Job drawing, mm, ordinate dimensions from the low corner. One solid piece. A direction names the side the tool comes from. Give positions to 0.01 mm unless a question says otherwise; leave off trailing zeros. Order: outer loops, then holes, each group sorted by start corner. A loop starts at its lowest first (then second) coordinate and runs counter-clockwise, first axis right, second up. Notation, with made-up numbers: M 14.25,70 L 28.25,70 A17 ccw 28.25,101 Z; hole C -13,87.5 d5. An arc over 180 degrees is marked long. Use CSV: the item, a comma, the result in double quotes. Start each with the question number.
Item 1: Wall check: line 1 along Z through (x, y) = (24, 6.25); line 2 along X through (y, z) = (16.5, 6.5); line 3 along Y through (x, z) = (31, 18.25). Give the ranges that are in metal, low to high.
Item 2: Band-saw the part on D-D on z = 12.5. Write the cut outline in (x, y), plus the area to 3 significant figures.
Item 3: Band-saw the part on A-A on x = 20. Write the cut outline in (y, z), plus the area to 3 significant figures.
Item 4: Two-plate mould, pull along X, no slides. Class the marked faces 1, 2 and 3: pulls with the +X half, pulls with the -X half, needs draft (parallel to the pull), parting line crosses it, or undercut.
Item 5: Which spindle directions (+Z, -Z, +X, -X, +Y, -Y) get a long thin tool onto all of the face, cutting with end or side? Do the marked faces 4 and 5. Say none if no direction does.
Item 6: Band-saw the part on B-B on z = 18. Write the cut outline in (x, y).
Item 7: Band-saw the part on C-C on y = 9.5. Write the cut outline in (x, z), plus the area to 3 significant figures.
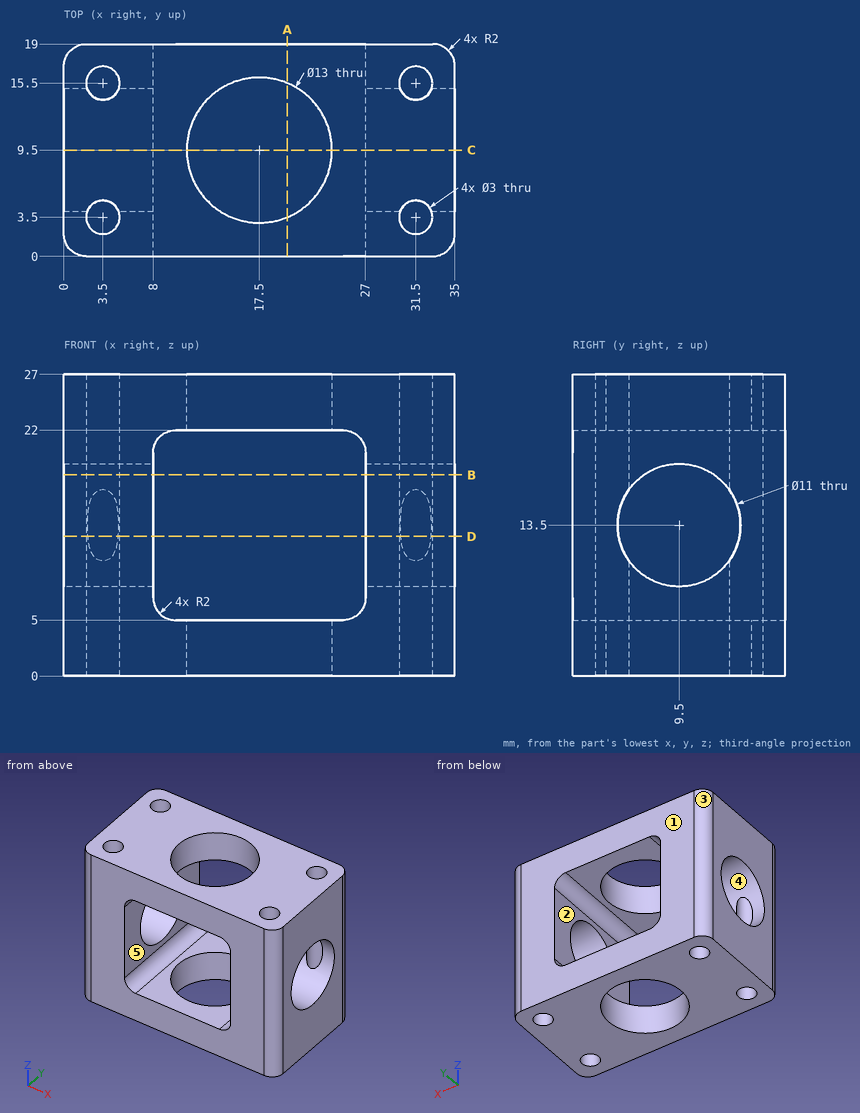
Model answer:
1,line 1,"z = 0 to 5, 22 to 27"
1,line 2,"x = 0 to 2.38, 4.62 to 8.06, 26.94 to 30.38, 32.62 to 35"
1,line 3,"y = 0 to 2.09, 4.91 to 6.73, 12.27 to 14.09, 16.91 to 19"
2,outline,"M 0,2 A2 ccw 2,0 L 8,0 L 8,4.09 L 4.88,4.09 A1.5 cw long 2.12,4.09 L 0,4.09 Z; M 0,14.91 L 2.12,14.91 A1.5 cw long 4.88,14.91 L 8,14.91 L 8,19 L 2,19 A2 ccw 0,17 Z; M 27,0 L 33,0 A2 ccw 35,2 L 35,4.09 L 32.88,4.09 A1.5 cw long 30.12,4.09 L 27,4.09 Z; M 27,14.91 L 30.12,14.91 A1.5 cw long 32.88,14.91 L 35,14.91 L 35,17 A2 ccw 33,19 L 27,19 Z"
2,area,"106 mm^2"
3,outline,"M 0,0 L 3.5,0 L 3.5,5 L 0,5 Z; M 0,22 L 3.5,22 L 3.5,27 L 0,27 Z; M 15.5,0 L 19,0 L 19,5 L 15.5,5 Z; M 15.5,22 L 19,22 L 19,27 L 15.5,27 Z"
3,area,"70.0 mm^2"
4,face 1,"needs draft"
4,face 2,"undercut"
4,face 3,"pulls with the -X half"
5,face 4,"+X, -X"
5,face 5,"+Y, -Y"
6,outline,"M 0,2 A2 ccw 2,0 L 8,0 L 8,6.34 L 0,6.34 Z; M 0,12.66 L 8,12.66 L 8,19 L 2,19 A2 ccw 0,17 Z; M 27,0 L 33,0 A2 ccw 35,2 L 35,6.34 L 27,6.34 Z; M 27,12.66 L 35,12.66 L 35,17 A2 ccw 33,19 L 27,19 Z; hole C 3.5,3.5 d3; hole C 3.5,15.5 d3; hole C 31.5,3.5 d3; hole C 31.5,15.5 d3"
7,outline,"M 0,0 L 11,0 L 11,5 L 10,5 A2 cw 8,7 L 8,8 L 0,8 Z; M 0,19 L 8,19 L 8,20 A2 cw 10,22 L 11,22 L 11,27 L 0,27 Z; M 24,0 L 35,0 L 35,8 L 27,8 L 27,7 A2 cw 25,5 L 24,5 Z; M 24,22 L 25,22 A2 cw 27,20 L 27,19 L 35,19 L 35,27 L 24,27 Z"
7,area,"319 mm^2"
